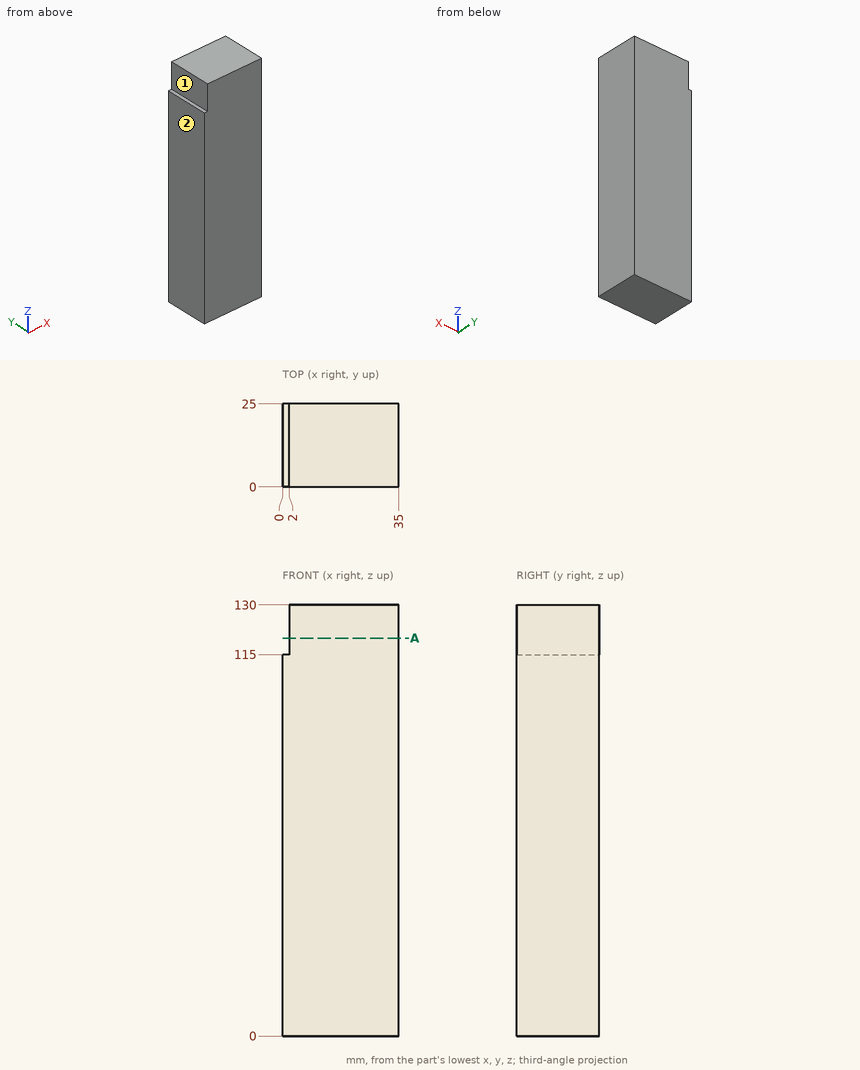
Job drawing, mm, ordinate dimensions from the low corner. One solid piece. A direction names the side the tool comes from. Round coordinates to 2 decimals unless told otherwise and drop trailing zeros. Order: outer loops, then holes, each group sorted by start corner. A loop starts at its lowest first (then second) coordinate and runs counter-clockwise, first axis right, second up. Notation, with made-up numbers: (48, 46) - (99, 46) arc R17 ccw to (99, 55) - close; hole circle Ø2 at (58.25, 16). An arc over 180 degrees is marked (long way). Use CSV: the item, a comma, the result in double quotes. Start each with the question number.
1) Saw through at A-A (z = 120). List the corners of the cut face in (x, y).
2) Wall check: L1, parallel to X at y = 9, z = 119. Give the ranges that are in metal, low to high. Write a range as [from, to].
3) Pin check, flat tips, straight feed: pin 1 Ø1 at (x, y) = (0.5, 10.5) entering from +Z; pin 2 Ø4.5 at (y, z) = (12, 126) entering from -X. Stop position of each tip, or through.
4) Tool access for the marked faces 1 and 2: list every direction of +Z, -Z, +X, -X, +Y, -Y with a clear straight run to the whole face (end or side of a thin tool).
Values follow:
1,outline,"(2, 0) - (35, 0) - (35, 25) - (2, 25) - close"
2,L1,"x = [2, 35]"
3,pin 1,"stops at z = 115"
3,pin 2,"stops at x = 2"
4,face 1,"+Z, -X, +Y, -Y"
4,face 2,"+Z, -Z, -X, +Y, -Y"
